Autodesk Inventor part; units mm, degrees
ref_plane "YZ Plane" through (0, 0, 0) normal (1, 0, 0) x (0, 1, 0)
ref_plane "XZ Plane" through (0, 0, 0) normal (0, 1, 0) x (-1, 0, 0)
ref_plane "XY Plane" through (0, 0, 0) normal (0, 0, 1) x (1, 0, 0)
sketch "Sketch1" plane through (0, 0, 0) normal (0, 0, 1) x (1, 0, 0)
  line L0 (0, 0) -> (6.175, 0)
  line L1 (9.75, -2.064) -> (9.75, -4.7)
  line L2 (5.75, -5.3) -> (4, -5.3)
  line L3 (4, -5.3) -> (4, -35.3)
  line L4 (4, -35.3) -> (0, -35.3)
  line L5 (0, -35.3) -> (0, 0)
  line L6 (5.75, -5.3) -> (5.75, -4.7)
  line L7 (5.75, -4.7) -> (9.75, -4.7)
  line L8 (6.175, 0) -> (9.75, -2.064)
  dimension "d0" = 19.5
  dimension "d1" = 8
  dimension "d3" = 30
  dimension "d4" = 11.5
  dimension "d5" = 0.6
  dimension "d22" = 30
  dimension "d23" = 12.35
  dimension "d24" = 5.3
revolve "Revolution1" add sketch "Sketch1" angle 360 about axis through (0, -35.3, 0) along (0, 1, 0)
sketch "Sketch2" plane through (0, 0, 0) normal (0, 1, 0) x (1, 0, 0)
  line L0 (0, -7.5056) -> (-6.5, -3.7528)
  line L1 (-6.5, -3.7528) -> (-6.5, 3.7528)
  line L2 (-6.5, 3.7528) -> (0, 7.5056)
  line L3 (0, 7.5056) -> (6.5, 3.7528)
  line L4 (6.5, 3.7528) -> (6.5, -3.7528)
  line L5 (6.5, -3.7528) -> (0, -7.5056)
  circle A0 centre (0, 0) radius 9.75
  point P0 (0, 0)
  point P1 (0, 0)
  dimension "d25" = 13
extrude "Extrusion1" cut sketch "Sketch2" against normal blind 5.3
thread "Thread1"
chamfer "Chamfer1" distance 0.6667 angle 45 1 edges at (-4, -35.3, 0)
equation "\"d0\" = 1.5 * S_"
equation "\"d1\" = d1_"
equation "\"d3\" = L"
equation "\"d4\" = dw"
equation "\"d5\" = hw"
equation "\"d23\" = 0.95 * S_"
equation "\"d24\" = k"
equation "\"d14\" = b"
equation "\"d16\" = 0.0833333 * d"
equation "\"d25\" = S_"
equation "\"d26\" = k"
equation "\"d\" = 8"
equation "\"d1_\" = 8"
equation "\"S_\" = 13"
equation "\"k\" = 5.3"
equation "\"e\" = 14.2"
equation "\"L\" = 30"
equation "\"b\" = 22"
equation "\"Grip_Length\" = 8"
equation "\"dw\" = 11.5"
equation "\"hw\" = 0.6"
properties part number "Bolt A M8-6g×30(S13) GOST 7798-70" material "Steel, Mild"
Model file for the job. Use its own axes, mm. A direction names the side the tool comes from. Coordinates: 2 decimals unless noted, no trailing zeros. Loops run counter-clockwise (first coordinate to the right, second up) from the corner with the lowest first, then second, coordinate; pieces in that order, holes last. Notation, with made-up numbers: (-21, -10) - (-14, -10) arc R13 ccw to (-14, 9) - close; hole circle Ø4 at (58.5, 74). An arc over 180 degrees is marked (long way). Write item = value, one per line. Start each with the question number.
Item 1: Saw through at B-B, the plane y = -13. List the corners of the cut face in (x, z), then the cut area to 3 significant figures.
Item 2: Wall check: probe 1 along X at (y, z) = (-6, 0); probe 2 along Y at (x, z) = (1.5, 4); probe 3 along Y at (x, z) = (-0.75, -3.25). Give the ranges that are in metal, low to high. Write a range as [from, to].
Item 3: Saw through at A-A, the plane z = 0. List the corners of the cut face in (x, y) (3 decimals).
Item 4: Drop flat-ended pins along their axis: pin 1 Ø6 at (y, z) = (-16, -3.5) entering from -X; pin 2 Ø4 at (x, y) = (-5, -17.5) entering from -Z; pin 3 Ø2 at (x, y) = (-3, -24) entering from +Z. Give the stop position or say it passes through.
Item 5: 3-axis set-ups, long thin cutter, end or side, ignore diameter. For faces 1 (the face through (-0.75, -5, -5.7)), 2 (the face through (0, 0, 0)): which of +Z, -Z, +X, -X, +Y, -Y reach the whole face in a straight line?
Answers:
q1.outline = circle Ø8 at (0, 0)
q1.area = 50.3 mm2
q2.probe_1 = [-4, 4]
q2.probe_2 = [-5.3, 0]
q2.probe_3 = [-35.3, 0]
q3.outline = (-6.5, -4.7) - (-5.75, -4.7) - (-5.75, -5.3) - (-4, -5.3) - (-4, -34.633) - (-3.333, -35.3) - (3.333, -35.3) - (4, -34.633) - (4, -5.3) - (5.75, -5.3) - (5.75, -4.7) - (6.5, -4.7) - (6.5, -0.188) - (6.175, 0) - (-6.175, 0) - (-6.5, -0.188) - close
q4.pin_1 = -3.97
q4.pin_2 = -2.65
q4.pin_3 = 3.46
q5.face_1 = -Y
q5.face_2 = +Z, -Z, +X, -X, +Y
